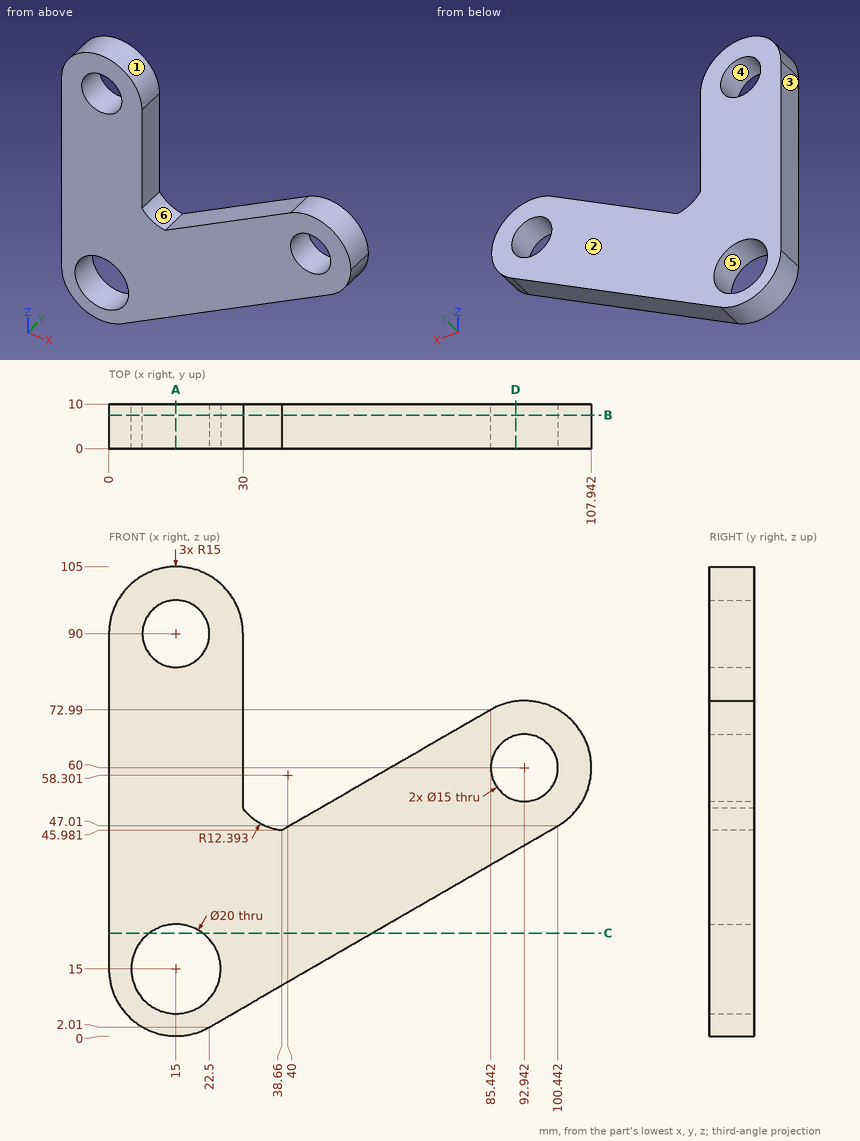
The figure shows three views and two pictorial views of one solid part (mm, origin at its lowest corner). Answer the questions. A direction names the side the tool comes from. Round coordinates to 2 decimals unless told otherwise and drop trailing zeros. Order: outer loops, then holes, each group sorted by start corner. A loop starts at its lowest first (then second) coordinate and runs counter-clockwise, first axis right, second up. Notation, with made-up numbers: M 37,-28 L 54,-28 A20 cw 54,7 Z; hole C 0.25,77.25 d11. An arc over 180 degrees is marked long. Put each result on its own line as item: value. Start each with the question number.
Q1. Section A-A, the plane x = 15 is taken. Write down the section's boundary in (y, z), and give its area (3 significant figures).
Q2. For a pull along X with two mould halves and no side action, classify the marked faces 1, 2, 3 and 4 as pulls with the +X half, pulls with the -X half, needs draft (parallel to the pull), parting line crosses it, or undercut.
Q3. Section D-D, the plane x = 91 is taken. Write down the section's boundary in (y, z).
Q4. Section B-B, the plane y = 7.5 is taken. Write down the section's boundary in (x, z).
Q5. Flat-ended cylindrical pins translate along their axes: pin 1 (1.5 mm diameter, centred on x = 79, z = 56, fed in from -Y); pin 2 (3 mm diameter, centred on y = 4.5, z = 74, fed in from +X) (1 decimal); pin 3 (1.5 mm diameter, centred on x = 96, y = 3, fed in from +Z); pin 4 (1 mm diameter, centred on x = 81.5, y = 2.5, fed in from -Z) (1 decimal). Find the tip coordinate at first contact, or state that the pin passes through.
Q6. A tool of negligible diameter and unlimited length cuts with its end or side. For the marked faces 5 and 6, from which of +Z, -Z, +X, -X, +Y, -Y can it reach the whole face along a straight path? Write none if from no direction.
Q7. Section C-C, the plane z = 23 is taken. Write down the section's boundary in (x, y).
Q8. Straight lines are drawn through the part: L1, parallel to Z at x = 15, y = 7; L2, parallel to Z at x = 13, y = 5.5 (1 decimal); L3, parallel to X at y = 1, z = 89.5. For each, find the intervals that lie inside material, in ascending order. Write a range as [from, to].
Findings below:
1. outline: M 0,0 L 10,0 L 10,5 L 0,5 Z; M 0,25 L 10,25 L 10,82.5 L 0,82.5 Z; M 0,97.5 L 10,97.5 L 10,105 L 0,105 Z
1. area: 700 mm^2
2. face 1: parting line crosses it
2. face 2: needs draft
2. face 3: pulls with the -X half
2. face 4: undercut
3. outline: M 0,41.56 L 10,41.56 L 10,52.76 L 0,52.76 Z; M 0,67.24 L 10,67.24 L 10,74.87 L 0,74.87 Z
4. outline: M 0,15 A15 ccw 22.5,2.01 L 100.44,47.01 A15 ccw 85.44,72.99 L 38.66,45.98 A12.39 cw 30,50.98 L 30,90 A15 ccw 0,90 Z; hole C 15,15 d20; hole C 15,90 d15; hole C 92.94,60 d15
5. pin 1: stops at y = 0
5. pin 2: stops at x = 101.2
5. pin 3: stops at z = 74.82
5. pin 4: stops at z = 35.8
6. face 5: +Y, -Y
6. face 6: +Z, +Y, -Y
7. outline: M 0,0 L 9,0 L 9,10 L 0,10 Z; M 21,0 L 58.86,0 L 58.86,10 L 21,10 Z
8. L1: z = [0, 5], [25, 82.5], [97.5, 105]
8. L2: z = [0.1, 5.2], [24.8, 82.8], [97.2, 104.9]
8. L3: x = [0, 7.52], [22.48, 30]
